from build123d import *

# Parameters (mm, degrees)
F_10_MM_DEEP_HAT_SECTION_DEPTH = 68


with BuildPart() as part:
    # 10 mm deep hat section profile → 10 mm deep hat section (new body)
    with BuildSketch(Plane.XY):
        Polygon((-8, 7), (-4, 7), (-4, 17), (4, 17), (4, 7), (8, 7), (8, 8), (5, 8), (5, 18), (-5, 18), (-5, 8), (-8, 8), align=None)
    extrude(amount=F_10_MM_DEEP_HAT_SECTION_DEPTH)


solid = part.part
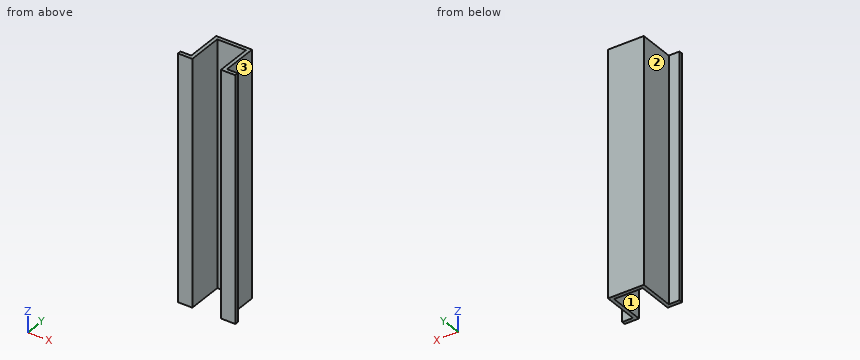
The model under review builds one solid part; all positions refer to its coordinate system, in mm. Face numbers are marked on the shaded views. A direction names the side the tool comes from. Give positions to 0.01 mm unless a question says otherwise; leave off trailing zeros. Loops run counter-clockwise (first coordinate to the right, second up) from the corner with the lowest first, then second, coordinate; pieces in that order, holes last. Notation, with made-up numbers: (-27, 72) -> (-17, 72) arc R11 ccw to (-17, 84) -> close; hole circle Ø10 at (80, 19). An arc over 180 degrees is marked (long way). Answer as a JSON object with one key per item and string values. Group by question number.
Q1. Wall thickness on line 1 along X through (y, z) = (11.5, 57); line 2 along Y through (x, z) = (-7, 35); line 3 along Y through (x, z) = (-1.5, 63): over which ranges is each line inside the solid? List them lowest first.
Q2. Take a section at A-A (y = 15.5). Write out the cut boundary in (x, z), plus the area to 3 significant figures.
Q3. Take a section at C-C (x = 1.5). Write out the cut boundary in (y, z), plus the area to 3 significant figures.
Q4. Tool access review of the marked faces 1, 2 and 3: name each direction out of +Z, -Z, +X, -X, +Y, -Y from which nothing blocks a thin tool from reaching the whole face with its end or side.
Q5. Insertion check: pin 1 (3.5 mm diameter, centred on x = 7, z = 28.5, fed in from +Y); pin 2 (3 mm diameter, centred on y = 11.5, z = 41, fed in from -X); pin 3 (2.5 mm diameter, centred on x = -0.5, z = 29.5, fed in from -Y). Each pin has a flat end and moves straight along its axis. Give the tip position at first contact, or say it passes through.
Q6. Take a section at B-B (z = 6). Write out the cut boundary in (x, y).
Answer below:
{
 "1": {"line 1": "x = -5 to -4, 4 to 5", "line 2": "y = 7 to 8", "line 3": "y = 17 to 18"},
 "2": {"outline": "(-5, 0) -> (-4, 0) -> (-4, 68) -> (-5, 68) -> close; (4, 0) -> (5, 0) -> (5, 68) -> (4, 68) -> close", "area": "136 mm2"},
 "3": {"outline": "(17, 0) -> (18, 0) -> (18, 68) -> (17, 68) -> close", "area": "68.0 mm2"},
 "4": {"face 1": "+Z, -Z, -Y", "face 2": "+Z, -Z, -X, +Y", "face 3": "+Z, -Z, +X, +Y"},
 "5": {"pin 1": "stops at y = 8", "pin 2": "stops at x = -5", "pin 3": "stops at y = 17"},
 "6": {"outline": "(-8, 7) -> (-4, 7) -> (-4, 17) -> (4, 17) -> (4, 7) -> (8, 7) -> (8, 8) -> (5, 8) -> (5, 18) -> (-5, 18) -> (-5, 8) -> (-8, 8) -> close"}
}
